Input: part model. Units: mm. Frame: model coordinates. A direction names the side the tool comes from. Round coordinates to 2 decimals unless told otherwise and drop trailing zeros. Use CSV: the item, a comma, the result in double quotes. Start each with the question number.
1. Material intervals for probe 1 along Y at (x, z) = (0, -70); probe 2 along Y at (x, z) = (-13.5, -158.5); probe 3 along X at (y, z) = (11, -189), sorted ascending. Write a range as from..to.
2. Pull-direction query (Y, two-part tool) for faces 1 (the flat face through (5, 0, 0)), 2 (the flat face through (-7.604, -10.496, -150.266)), 3 (the flat face through (7.67, -10.56, -150.27)), 4 (the flat face through (12, -19.05, -150)); classes: +Y half, -Y half, draft (parallel to the pull), parting line (faces both ways), or undercut.
3. Access query for faces 5 (the flat face through (19.05, 12, -150)), 6 (the flat face through (10.546, 7.691, -150.266)). Directions: +Z, -Z, +X, -X, +Y, -Y. A direction counts if a zero-diameter tool reaches every point of the face in a straight line with its end or side. Return the directions, or none.
4. Pin query (flat end, axial travel): P1, Ø1.2, axis at y = -0.5, z = -111.5, coming from the +X side; P2, Ø6, axis at y = 0, z = -34.5, coming from the +X side; P3, Ø0.8, axis at x = -17, z = -120, coming from the +Y side. Return the tip coordinate at first contact, or that it passes through.
```python
from build123d import *

# Parameters (mm, degrees)
SKETCH1_R = 3.3274


with BuildPart() as part:
    # Sweep4: sweep along a path in Sketch2
    with BuildLine(Plane(origin=(0, 0, 0), x_dir=(1, 0, 0), z_dir=(0, 1, 0))) as sweep4_path:
        Line((0, 304.8), (0, 275))
        Line((0, 275), (0, 0))
    # Sketch1 → Sweep4 (sweep)
    with BuildSketch(Plane(origin=(0, 0, -304.8), x_dir=(-1, 0, 0), z_dir=(0, 0, -1))):
        with BuildLine():
            Line((14.327719201, 19.050000003), (9.498178698, 19.050000003))
            ThreePointArc((9.498178698, 19.050000003), (8.736178698, 18.288000003), (7.974178698, 19.050000003))
            Line((7.974178698, 19.050000003), (5.61761756, 19.050000003))
            ThreePointArc((5.61761756, 19.050000003), (4.519044055, 18.594955959), (4.06400001, 17.496382454))
            Line((4.06400001, 17.496382454), (4.06400001, 16.539617563))
            ThreePointArc((4.06400001, 16.539617563), (4.519044055, 15.441044058), (5.61761756, 14.986000013))
            Line((5.61761756, 14.986000013), (9.38530001, 14.986000013))
            ThreePointArc((9.38530001, 14.986000013), (10.022898195, 14.721898198), (10.28700001, 14.084300013))
            Line((10.28700001, 14.084300013), (10.28700001, 13.552357144))
            ThreePointArc((10.28700001, 13.552357144), (10.218362397, 13.207292006), (10.022898979, 12.914759744))
            Line((10.022898979, 12.914759744), (5.252158118, 8.144007146))
            ThreePointArc((5.252158118, 8.144007146), (3.715177385, 7.117027402), (1.902183988, 6.756400013))
            Line((1.902183988, 6.756400013), (-1.902183965, 6.756400013))
            ThreePointArc((-1.902183965, 6.756400013), (-3.715177361, 7.117027401), (-5.252158094, 8.144007145))
            Line((-5.252158094, 8.144007145), (-10.022898959, 12.914759744))
            ThreePointArc((-10.022898959, 12.914759744), (-10.218362376, 13.207292006), (-10.28699999, 13.552357144))
            Line((-10.28699999, 13.552357144), (-10.28699999, 14.084300013))
            ThreePointArc((-10.28699999, 14.084300013), (-10.022898174, 14.721898198), (-9.38529999, 14.986000013))
            Line((-9.38529999, 14.986000013), (-5.617617539, 14.986000013))
            ThreePointArc((-5.617617539, 14.986000013), (-4.519044035, 15.441044058), (-4.06399999, 16.539617563))
            Line((-4.06399999, 16.539617563), (-4.06399999, 17.496382454))
            ThreePointArc((-4.06399999, 17.496382454), (-4.519044035, 18.594955959), (-5.617617539, 19.050000003))
            Line((-5.617617539, 19.050000003), (-7.974178709, 19.050000003))
            ThreePointArc((-7.974178709, 19.050000003), (-8.736178709, 18.288000003), (-9.498178709, 19.050000003))
            Line((-9.498178709, 19.050000003), (-14.327719212, 19.050000003))
            ThreePointArc((-14.327719212, 19.050000003), (-15.087603125, 18.231251135), (-15.847487045, 19.049999996))
            ThreePointArc((-15.847487045, 19.049999996), (-18.120176306, 18.120192065), (-19.050000001, 15.847509253))
            ThreePointArc((-19.050000001, 15.847509253), (-18.231251012, 15.087625373), (-19.049999993, 14.327741484))
            Line((-19.049999993, 14.327741484), (-19.049999993, 9.49609147))
            ThreePointArc((-19.049999993, 9.49609147), (-18.231250986, 8.736207564), (-19.049999993, 7.976323658))
            Line((-19.049999993, 7.976323658), (-19.049999993, 5.617617549))
            ThreePointArc((-19.049999993, 5.617617549), (-18.594955948, 4.519044045), (-17.496382444, 4.064))
            Line((-17.496382444, 4.064), (-16.539617542, 4.064))
            ThreePointArc((-16.539617542, 4.064), (-15.441044038, 4.519044045), (-14.985999993, 5.617617549))
            Line((-14.985999993, 5.617617549), (-14.985999993, 9.385342517))
            ThreePointArc((-14.985999993, 9.385342517), (-14.721898178, 10.022940702), (-14.084299993, 10.287042517))
            Line((-14.084299993, 10.287042517), (-13.516042079, 10.287042517))
            ThreePointArc((-13.516042079, 10.287042517), (-13.170975915, 10.218404479), (-12.87844311, 10.022939917))
            Line((-12.87844311, 10.022939917), (-8.147580073, 5.292065242))
            ThreePointArc((-8.147580073, 5.292065242), (-7.117955872, 3.751120652), (-6.756399993, 1.933453584))
            Line((-6.756399993, 1.933453584), (-6.756399993, -1.933453584))
            ThreePointArc((-6.756399993, -1.933453584), (-7.117955872, -3.751120652), (-8.147580073, -5.292065242))
            Line((-8.147580073, -5.292065242), (-12.87844311, -10.022939917))
            ThreePointArc((-12.87844311, -10.022939917), (-13.170975915, -10.218404479), (-13.516042079, -10.287042517))
            Line((-13.516042079, -10.287042517), (-14.084299993, -10.287042517))
            ThreePointArc((-14.084299993, -10.287042517), (-14.721898178, -10.022940702), (-14.985999993, -9.385342517))
            Line((-14.985999993, -9.385342517), (-14.985999993, -5.617617549))
            ThreePointArc((-14.985999993, -5.617617549), (-15.441044038, -4.519044045), (-16.539617542, -4.064))
            Line((-16.539617542, -4.064), (-17.496382444, -4.064))
            ThreePointArc((-17.496382444, -4.064), (-18.594955948, -4.519044045), (-19.049999993, -5.617617549))
            Line((-19.049999993, -5.617617549), (-19.049999993, -7.97631849))
            ThreePointArc((-19.049999993, -7.97631849), (-18.231250986, -8.736202396), (-19.049999993, -9.496086301))
            Line((-19.049999993, -9.496086301), (-19.049999993, -14.327742909))
            ThreePointArc((-19.049999993, -14.327742909), (-18.231250983, -15.08762681), (-19.049999984, -15.847510721))
            ThreePointArc((-19.049999984, -15.847510721), (-18.120175688, -18.120192657), (-15.847486815, -19.049999997))
            ThreePointArc((-15.847486815, -19.049999997), (-15.087602925, -18.231251148), (-14.327719025, -19.049999987))
            Line((-14.327719025, -19.049999987), (-9.496062438, -19.049999987))
            ThreePointArc((-9.496062438, -19.049999987), (-8.736178522, -18.231251122), (-7.976294605, -19.049999987))
            Line((-7.976294605, -19.049999987), (-5.617617539, -19.049999987))
            ThreePointArc((-5.617617539, -19.049999987), (-4.519044035, -18.594955942), (-4.06399999, -17.496382437))
            Line((-4.06399999, -17.496382437), (-4.06399999, -16.539617536))
            ThreePointArc((-4.06399999, -16.539617536), (-4.519044035, -15.441044031), (-5.617617539, -14.985999987))
            Line((-5.617617539, -14.985999987), (-9.38529999, -14.985999987))
            ThreePointArc((-9.38529999, -14.985999987), (-10.022898174, -14.721898171), (-10.28699999, -14.084299987))
            Line((-10.28699999, -14.084299987), (-10.28699999, -13.552357118))
            ThreePointArc((-10.28699999, -13.552357118), (-10.218362376, -13.207291979), (-10.022898959, -12.914759717))
            Line((-10.022898959, -12.914759717), (-5.252158094, -8.144007118))
            ThreePointArc((-5.252158094, -8.144007118), (-3.715177361, -7.117027375), (-1.902183965, -6.756399987))
            Line((-1.902183965, -6.756399987), (1.902183988, -6.756399987))
            ThreePointArc((1.902183988, -6.756399987), (3.715177385, -7.117027375), (5.252158118, -8.144007119))
            Line((5.252158118, -8.144007119), (10.022898979, -12.914759717))
            ThreePointArc((10.022898979, -12.914759717), (10.218362397, -13.207291979), (10.28700001, -13.552357118))
            Line((10.28700001, -13.552357118), (10.28700001, -14.084299987))
            ThreePointArc((10.28700001, -14.084299987), (10.022898195, -14.721898171), (9.38530001, -14.985999987))
            Line((9.38530001, -14.985999987), (5.61761756, -14.985999987))
            ThreePointArc((5.61761756, -14.985999987), (4.519044055, -15.441044031), (4.06400001, -16.539617536))
            Line((4.06400001, -16.539617536), (4.06400001, -17.496382437))
            ThreePointArc((4.06400001, -17.496382437), (4.519044055, -18.594955942), (5.61761756, -19.049999987))
            Line((5.61761756, -19.049999987), (7.976294626, -19.049999987))
            ThreePointArc((7.976294626, -19.049999987), (8.736178543, -18.231251122), (9.496062459, -19.049999987))
            Line((9.496062459, -19.049999987), (14.327719046, -19.049999987))
            ThreePointArc((14.327719046, -19.049999987), (15.087602959, -18.231251119), (15.847486878, -19.04999998))
            ThreePointArc((15.847486878, -19.04999998), (18.12017574, -18.120192611), (19.050000007, -15.847510662))
            ThreePointArc((19.050000007, -15.847510662), (18.231250911, -15.087626785), (19.050000007, -14.327742909))
            Line((19.050000007, -14.327742909), (19.050000007, -9.496086301))
            ThreePointArc((19.050000007, -9.496086301), (18.231251003, -8.736202395), (19.050000007, -7.976318489))
            Line((19.050000007, -7.976318489), (19.050000007, -5.617617549))
            ThreePointArc((19.050000007, -5.617617549), (18.594955962, -4.519044045), (17.496382458, -4.064))
            Line((17.496382458, -4.064), (16.539617556, -4.064))
            ThreePointArc((16.539617556, -4.064), (15.441044052, -4.519044045), (14.986000007, -5.617617549))
            Line((14.986000007, -5.617617549), (14.986000007, -9.385342517))
            ThreePointArc((14.986000007, -9.385342517), (14.721898191, -10.022940702), (14.084300007, -10.287042517))
            Line((14.084300007, -10.287042517), (13.516042095, -10.287042517))
            ThreePointArc((13.516042095, -10.287042517), (13.170975932, -10.218404479), (12.878443126, -10.022939918))
            Line((12.878443126, -10.022939918), (8.147580087, -5.292065243))
            ThreePointArc((8.147580087, -5.292065243), (7.117955886, -3.751120653), (6.756400007, -1.933453584))
            Line((6.756400007, -1.933453584), (6.756400007, 1.933453584))
            ThreePointArc((6.756400007, 1.933453584), (7.117955886, 3.751120653), (8.147580087, 5.292065243))
            Line((8.147580087, 5.292065243), (12.878443126, 10.022939918))
            ThreePointArc((12.878443126, 10.022939918), (13.170975932, 10.218404479), (13.516042095, 10.287042517))
            Line((13.516042095, 10.287042517), (14.084300007, 10.287042517))
            ThreePointArc((14.084300007, 10.287042517), (14.721898191, 10.022940702), (14.986000007, 9.385342517))
            Line((14.986000007, 9.385342517), (14.986000007, 5.617617549))
            ThreePointArc((14.986000007, 5.617617549), (15.441044052, 4.519044045), (16.539617556, 4.064))
            Line((16.539617556, 4.064), (17.496382458, 4.064))
            ThreePointArc((17.496382458, 4.064), (18.594955962, 4.519044045), (19.050000007, 5.617617549))
            Line((19.050000007, 5.617617549), (19.050000007, 7.976323659))
            ThreePointArc((19.050000007, 7.976323659), (18.231251003, 8.736207565), (19.050000007, 9.496091471))
            Line((19.050000007, 9.496091471), (19.050000007, 14.327741484))
            ThreePointArc((19.050000007, 14.327741484), (18.231251061, 15.087625385), (19.049999988, 15.847509306))
            ThreePointArc((19.049999988, 15.847509306), (18.120176278, 18.120192088), (15.847487034, 19.050000003))
            ThreePointArc((15.847487034, 19.050000003), (15.087603117, 18.231251142), (14.327719201, 19.050000003))
        make_face()
        Circle(SKETCH1_R, mode=Mode.SUBTRACT)
    sweep(path=sweep4_path.line)


solid = part.part
```
Established:
1,probe 1,"y = -6.76..-3.33, 3.33..6.76"
1,probe 2,"y = -19.05..-10.29, 10.29..19.05"
1,probe 3,"x = -19.05..-8.11, 8.11..19.05"
2,face 1,"draft"
2,face 2,"undercut"
2,face 3,"undercut"
2,face 4,"-Y half"
3,face 5,"+Z, -Z, +X, +Y, -Y"
3,face 6,"+Z, -Z"
4,P1,"stops at x = 6.76"
4,P2,"stops at x = 6.88"
4,P3,"stops at y = 18.97"
